```python
from build123d import *

# Parameters (mm, degrees)
SKETCH1_W          = 100
SKETCH1_H          = 62
BASE_FLANGE1_DEPTH = 1.245
CUT_EXTRUDE7_DEPTH = 10
MOVE_FACE1_BY      = 5


# Sheet-metal steps are written as plain solids
with BuildPart() as part:
    # Sketch1 → Base-Flange1 (new body)
    with BuildSketch(Plane.XY):
        Rectangle(SKETCH1_W, SKETCH1_H)
    extrude(amount=-BASE_FLANGE1_DEPTH)

    # Sketch6 → Cut-Extrude7 (cut)
    with BuildSketch(Plane.XY):
        with BuildLine():
            Line((-43.645, 17.5), (-43.645, 13.511034779))
            ThreePointArc((-43.645, 13.511034779), (-41.605, 5), (-39.565, 13.511034779))
            Line((-39.565, 13.511034779), (-39.565, 17.5))
            ThreePointArc((-39.565, 17.5), (-41.605, 19.54), (-43.645, 17.5))
        make_face()
        with BuildLine():
            Line((39.565, 17.5), (39.565, 13.511034779))
            ThreePointArc((39.565, 13.511034779), (41.605, 5), (43.645, 13.511034779))
            Line((43.645, 13.511034779), (43.645, 17.5))
            ThreePointArc((43.645, 17.5), (41.605, 19.54), (39.565, 17.5))
        make_face()
        with BuildLine():
            Line((-43.645, -17.5), (-43.645, -21.488965221))
            ThreePointArc((-43.645, -21.488965221), (-41.605, -30), (-39.565, -21.488965221))
            Line((-39.565, -21.488965221), (-39.565, -17.5))
            ThreePointArc((-39.565, -17.5), (-41.605, -15.46), (-43.645, -17.5))
        make_face()
        with BuildLine():
            Line((39.565, -17.5), (39.565, -21.488965221))
            ThreePointArc((39.565, -21.488965221), (41.605, -30), (43.645, -21.488965221))
            Line((43.645, -21.488965221), (43.645, -17.5))
            ThreePointArc((43.645, -17.5), (41.605, -15.46), (39.565, -17.5))
        make_face()
    extrude(amount=-CUT_EXTRUDE7_DEPTH, mode=Mode.SUBTRACT)

    # Move Face1: a face moved inward by 5.0
    extrude(part.faces().sort_by_distance((0, 31, -0.6225))[0], amount=MOVE_FACE1_BY, dir=(0, -1, 0), mode=Mode.SUBTRACT)


solid = part.part
```
Here's how the part is built. I have some questions about the finished solid (model axes, mm). A direction names the side the tool comes from. Coordinates: 2 decimals unless noted, no trailing zeros. Write each loop counter-clockwise with the first axis right and the second up, starting at its lowest first coordinate (ties: lowest second). Pieces come first, ordered by that corner, then holes. Notation, with made-up numbers: (-16.5, 53) - (-6.5, 53) arc R28 cw to (-6.5, 83) - close; hole circle Ø6 at (54, 17). An arc over 180 degrees is marked (long way). One line per item, written item: value.
1) We'd pull the mould along Y, two halves only. Please class faces 3 (the flat face through (-1, -2, -1.245)), 4 (the cylindrical face through (-41.56, 19.54, -0.61)): pulls with the +Y half, pulls with the -Y half, needs draft (parallel to the pull), parting line crosses it, or undercut.
Model answer:
face 3: needs draft
face 4: undercut
2) I need wall thicknesses on line 1 along X through (y, z) = (9.5, -0.3) (3 decimals); line 2 along Y through (x, z) = (-41, -1.05); line 3 along X through (y, z) = (7.5, -0.7). Which ranges of each line are inside material? Lowest first, please.
Model answer:
line 1: x = -50 to -46.105, -37.105 to 37.105, 46.105 to 50
line 2: y = -31 to -29.96, -15.55 to 5.04, 19.45 to 26
line 3: x = -50 to -45.64, -37.57 to 37.57, 45.64 to 50
3) Suppose I cut it at C-C on x = 42. Write out the boundary of the cut face in (y, z) (3 decimals), and give its area (3 significant figures).
Model answer:
outline: (-31, -1.245) - (-29.983, -1.245) - (-29.983, 0) - (-31, 0) - close; (-15.499, -1.245) - (5.017, -1.245) - (5.017, 0) - (-15.499, 0) - close; (19.501, -1.245) - (26, -1.245) - (26, 0) - (19.501, 0) - close
area: 34.9 mm²
4) Suppose I cut it at A-A on y = -25.5. Write out the boundary of the cut face in (x, z) (3 decimals).
Model answer:
outline: (-50, -1.245) - (-46.105, -1.245) - (-46.105, 0) - (-50, 0) - close; (-37.105, -1.245) - (37.105, -1.245) - (37.105, 0) - (-37.105, 0) - close; (46.105, -1.245) - (50, -1.245) - (50, 0) - (46.105, 0) - close
5) I'm going to push flat-ended pins straight in: P1, Ø8, axis at x = 41.605, y = 9.5, coming from the -Z side; P2, Ø6, axis at x = 25, y = 8, coming from the +Z side. Where does each tip first touch, or does it pass through?
Model answer:
P1: passes through
P2: stops at z = 0
6) Suppose I cut it at B-B on z = -0.6. Write out the boundary of the cut face in (x, y) (3 decimals), and give its area (3 significant figures).
Model answer:
outline: (-50, -31) - (50, -31) - (50, 26) - (-50, 26) - close; hole (-43.645, -21.489) arc R4.5 ccw (long way) to (-39.565, -21.489) - (-39.565, -17.5) arc R2.04 ccw to (-43.645, -17.5) - close; hole (-43.645, 13.511) arc R4.5 ccw (long way) to (-39.565, 13.511) - (-39.565, 17.5) arc R2.04 ccw to (-43.645, 17.5) - close; hole (39.565, -21.489) arc R4.5 ccw (long way) to (43.645, -21.489) - (43.645, -17.5) arc R2.04 ccw to (39.565, -17.5) - close; hole (39.565, 13.511) arc R4.5 ccw (long way) to (43.645, 13.511) - (43.645, 17.5) arc R2.04 ccw to (39.565, 17.5) - close
area: 5,360 mm²
7) On a 3-axis mill with a long thin cutter (end or side, diameter ignored), from which of +Z, -Z, +X, -X, +Y, -Y can I reach the whole of each face in a straight line? I mean faces 1 (the cylindrical face through (41.65, 19.54, -0.61)), 2 (the flat face through (-1, -2, 0)). Say none if no direction works.
Model answer:
face 1: +Z, -Z
face 2: +Z, +X, -X, +Y, -Y
